from build123d import *

# Parameters (mm, degrees)
CYLINDER_R        = 3.25
CYLINDER_DEPTH    = 3.5
BOX017_W          = 43
BOX017_H          = 38
BOX017_DEPTH      = 0.5
BOX057_W          = 4
BOX057_H          = 8
BOX057_DEPTH      = 5.3
BOX001_W          = 4.5
BOX001_H          = 2.5
BOX001_DEPTH      = 5.3
BOX003_W          = 5.5
BOX003_H          = 3.5
BOX003_DEPTH      = 5.3
BOX002_W          = 53.8
BOX002_H          = 62.8
BOX002_DEPTH      = 5.3
BOX_W             = 56.3
BOX_H             = 64.25
BOX_DEPTH         = 5.3
BOX056_W          = 13.5
BOX056_H          = 1
BOX056_DEPTH      = 5
BOX041_W          = 44
BOX041_H          = 39
BOX041_DEPTH      = 0.5
BOX008_W          = 56.3
BOX008_H          = 39
BOX008_DEPTH      = 2
CHAMFER_SIZE      = 1.5
CYLINDER011_R     = 5
CYLINDER011_DEPTH = 0.5
BOX055_W          = 32
BOX055_H          = 10
BOX055_DEPTH      = 0.5
CYLINDER010_R     = 5
CYLINDER010_DEPTH = 0.5
BOX044_W          = 32
BOX044_H          = 12
BOX044_DEPTH      = 1
CYLINDER007_R     = 6
CYLINDER007_DEPTH = 1
CYLINDER006_R     = 6
CYLINDER006_DEPTH = 1
CYLINDER008_R     = 7
CYLINDER008_DEPTH = 1
BOX047_W          = 10
BOX047_H          = 1
BOX047_DEPTH      = 1
BOX049_W          = 10
BOX049_H          = 1
BOX049_DEPTH      = 1
BOX048_W          = 10
BOX048_H          = 1
BOX048_DEPTH      = 1
BOX046_W          = 10
BOX046_H          = 1
BOX046_DEPTH      = 1
BOX045_W          = 10
BOX045_H          = 1
BOX045_DEPTH      = 1
CYLINDER009_R     = 7
CYLINDER009_DEPTH = 1
BOX051_W          = 10
BOX051_H          = 1
BOX051_DEPTH      = 1
BOX054_W          = 10
BOX054_H          = 1
BOX054_DEPTH      = 1
BOX053_W          = 10
BOX053_H          = 1
BOX053_DEPTH      = 1
BOX052_W          = 10
BOX052_H          = 1
BOX052_DEPTH      = 1
BOX050_W          = 10
BOX050_H          = 1
BOX050_DEPTH      = 1
BOX010_W          = 10
BOX010_H          = 10
BOX010_DEPTH      = 10
BOX007_W          = 56.3
BOX007_H          = 25.25
BOX007_DEPTH      = 2


with BuildPart() as cylinder_magnet:
    # Cylinder → Cylinder (new body)
    with BuildSketch(Plane(origin=(52.8, 32.25, 3.7), x_dir=(0, 0, -1), z_dir=(1, 0, 0))):
        Circle(CYLINDER_R)
    extrude(amount=CYLINDER_DEPTH)


with BuildPart() as obj1:
    # Box017 → Box017 (new body)
    with BuildSketch(Plane(origin=(7.1, 8.5, 6.8), x_dir=(1, 0, 0), z_dir=(0, 0, 1))):
        with Locations((21.5, 19)):
            Rectangle(BOX017_W, BOX017_H)
    extrude(amount=BOX017_DEPTH)


with BuildPart() as cube_magnet_black:
    # Box057 → Box057 (new body)
    with BuildSketch(Plane(origin=(51.3, 28.25, 0), x_dir=(1, 0, 0), z_dir=(0, 0, 1))):
        with Locations((2, 4)):
            Rectangle(BOX057_W, BOX057_H)
    extrude(amount=BOX057_DEPTH)


with BuildPart() as cube_corner_inner:
    # Box001 → Box001 (new body)
    with BuildSketch(Plane(origin=(51.8, 61.75, 0), x_dir=(1, 0, 0), z_dir=(0, 0, 1))):
        with Locations((2.25, 1.25)):
            Rectangle(BOX001_W, BOX001_H)
    extrude(amount=BOX001_DEPTH)


with BuildPart() as cube_corner_outer:
    # Box003 → Box003 (new body)
    with BuildSketch(Plane(origin=(50.8, 60.75, 0), x_dir=(1, 0, 0), z_dir=(0, 0, 1))):
        with Locations((2.75, 1.75)):
            Rectangle(BOX003_W, BOX003_H)
    extrude(amount=BOX003_DEPTH)


with BuildPart() as cube_inner_base:
    # Box002 → Box002 (new body)
    with BuildSketch(Plane(origin=(1.25, 0, 0), x_dir=(1, 0, 0), z_dir=(0, 0, 1))):
        with Locations((26.9, 31.4)):
            Rectangle(BOX002_W, BOX002_H)
    extrude(amount=BOX002_DEPTH)


with BuildPart() as cut024:
    # Box → Box (new body)
    with BuildSketch(Plane.XY):
        with Locations((28.15, 32.125)):
            Rectangle(BOX_W, BOX_H)
    extrude(amount=BOX_DEPTH)

    # Cut: cut Cube(inner_base)
    add(cube_inner_base.part, mode=Mode.SUBTRACT)

    # Fusion: union Cube(corner_outer)
    add(cube_corner_outer.part)

    # Cut024: cut Cube(corner_inner)
    add(cube_corner_inner.part, mode=Mode.SUBTRACT)


with BuildPart() as cube_sd_card_cover:
    # Box056 → Box056 (new body)
    with BuildSketch(Plane(origin=(27.1, 63.25, -5), x_dir=(1, 0, 0), z_dir=(0, 0, 1))):
        with Locations((6.75, 0.5)):
            Rectangle(BOX056_W, BOX056_H)
    extrude(amount=BOX056_DEPTH)


with BuildPart() as obj2:
    # Box041 → Box041 (new body)
    with BuildSketch(Plane(origin=(6.6, 8, 6.8), x_dir=(1, 0, 0), z_dir=(0, 0, 1))):
        with Locations((22, 19.5)):
            Rectangle(BOX041_W, BOX041_H)
    extrude(amount=BOX041_DEPTH)


with BuildPart() as chamfer_body:
    # Box008 → Box008 (new body)
    with BuildSketch(Plane.XY.offset(5.3)):
        with Locations((28.15, 19.5)):
            Rectangle(BOX008_W, BOX008_H)
    extrude(amount=BOX008_DEPTH)

    # Chamfer
    chamfer_edges = [chamfer_body.edges().sort_by_distance(p)[0] for p in [
        (0, 19.5, 7.3),
        (56.3, 19.5, 7.3),
    ]]
    chamfer(chamfer_edges, length=CHAMFER_SIZE)


with BuildPart() as cylinder002_right_nintendo_inner:
    # Cylinder011 → Cylinder011 (new body)
    with BuildSketch(Plane(origin=(44.6, 55, 6.8), x_dir=(1, 0, 0), z_dir=(0, 0, 1))):
        Circle(CYLINDER011_R)
    extrude(amount=CYLINDER011_DEPTH)


with BuildPart() as cube_middle_nintendo_inner:
    # Box055 → Box055 (new body)
    with BuildSketch(Plane(origin=(12.6, 50, 6.8), x_dir=(1, 0, 0), z_dir=(0, 0, 1))):
        with Locations((16, 5)):
            Rectangle(BOX055_W, BOX055_H)
    extrude(amount=BOX055_DEPTH)


with BuildPart() as fusion033:
    # Cylinder010 → Cylinder010 (new body)
    with BuildSketch(Plane(origin=(12.6, 55, 6.8), x_dir=(1, 0, 0), z_dir=(0, 0, 1))):
        Circle(CYLINDER010_R)
    extrude(amount=CYLINDER010_DEPTH)

    # Fusion033: union Cylinder002(right_nintendo_inner), Cube(middle_nintendo_inner)
    add(cylinder002_right_nintendo_inner.part)
    add(cube_middle_nintendo_inner.part)


with BuildPart() as cube_middle_nintendo_outer:
    # Box044 → Box044 (new body)
    with BuildSketch(Plane(origin=(12.6, 49, 6.8), x_dir=(1, 0, 0), z_dir=(0, 0, 1))):
        with Locations((16, 6)):
            Rectangle(BOX044_W, BOX044_H)
    extrude(amount=BOX044_DEPTH)


with BuildPart() as cylinder002_right_nintendo_outer:
    # Cylinder007 → Cylinder007 (new body)
    with BuildSketch(Plane(origin=(44.6, 55, 6.8), x_dir=(1, 0, 0), z_dir=(0, 0, 1))):
        Circle(CYLINDER007_R)
    extrude(amount=CYLINDER007_DEPTH)


with BuildPart() as cylinder001_left_nintendo_outer:
    # Cylinder006 → Cylinder006 (new body)
    with BuildSketch(Plane(origin=(12.6, 55, 6.8), x_dir=(1, 0, 0), z_dir=(0, 0, 1))):
        Circle(CYLINDER006_R)
    extrude(amount=CYLINDER006_DEPTH)


with BuildPart() as cylinder001_left_nintendo_fin_cut:
    # Cylinder008 → Cylinder008 (new body)
    with BuildSketch(Plane(origin=(12.6, 55, 6.8), x_dir=(1, 0, 0), z_dir=(0, 0, 1))):
        Circle(CYLINDER008_R)
    extrude(amount=CYLINDER008_DEPTH)


with BuildPart() as box047:
    # Box047 → Box047 (new body)
    with BuildSketch(Plane(origin=(0, 54.5, 6.8), x_dir=(1, 0, 0), z_dir=(0, 0, 1))):
        with Locations((5, 0.5)):
            Rectangle(BOX047_W, BOX047_H)
    extrude(amount=BOX047_DEPTH)


with BuildPart() as box049:
    # Box049 → Box049 (new body)
    with BuildSketch(Plane(origin=(0, 58.5, 6.8), x_dir=(1, 0, 0), z_dir=(0, 0, 1))):
        with Locations((5, 0.5)):
            Rectangle(BOX049_W, BOX049_H)
    extrude(amount=BOX049_DEPTH)


with BuildPart() as box048:
    # Box048 → Box048 (new body)
    with BuildSketch(Plane(origin=(0, 56.5, 6.8), x_dir=(1, 0, 0), z_dir=(0, 0, 1))):
        with Locations((5, 0.5)):
            Rectangle(BOX048_W, BOX048_H)
    extrude(amount=BOX048_DEPTH)


with BuildPart() as box046:
    # Box046 → Box046 (new body)
    with BuildSketch(Plane(origin=(0, 52.5, 6.8), x_dir=(1, 0, 0), z_dir=(0, 0, 1))):
        with Locations((5, 0.5)):
            Rectangle(BOX046_W, BOX046_H)
    extrude(amount=BOX046_DEPTH)


with BuildPart() as cut009:
    # Box045 → Box045 (new body)
    with BuildSketch(Plane(origin=(0, 50.5, 6.8), x_dir=(1, 0, 0), z_dir=(0, 0, 1))):
        with Locations((5, 0.5)):
            Rectangle(BOX045_W, BOX045_H)
    extrude(amount=BOX045_DEPTH)

    # Fusion004: union Box047, Box049, Box048, Box046
    add(box047.part)
    add(box049.part)
    add(box048.part)
    add(box046.part)

    # Cut009: cut Cylinder001(left_nintendo_fin_cut)
    add(cylinder001_left_nintendo_fin_cut.part, mode=Mode.SUBTRACT)


with BuildPart() as cylinder002_right_nintendo_fin_cut:
    # Cylinder009 → Cylinder009 (new body)
    with BuildSketch(Plane(origin=(44.6, 55, 6.8), x_dir=(1, 0, 0), z_dir=(0, 0, 1))):
        Circle(CYLINDER009_R)
    extrude(amount=CYLINDER009_DEPTH)


with BuildPart() as box051:
    # Box051 → Box051 (new body)
    with BuildSketch(Plane(origin=(46.3, 54.5, 6.8), x_dir=(1, 0, 0), z_dir=(0, 0, 1))):
        with Locations((5, 0.5)):
            Rectangle(BOX051_W, BOX051_H)
    extrude(amount=BOX051_DEPTH)


with BuildPart() as box054:
    # Box054 → Box054 (new body)
    with BuildSketch(Plane(origin=(46.3, 52.5, 6.8), x_dir=(1, 0, 0), z_dir=(0, 0, 1))):
        with Locations((5, 0.5)):
            Rectangle(BOX054_W, BOX054_H)
    extrude(amount=BOX054_DEPTH)


with BuildPart() as box053:
    # Box053 → Box053 (new body)
    with BuildSketch(Plane(origin=(46.3, 56.5, 6.8), x_dir=(1, 0, 0), z_dir=(0, 0, 1))):
        with Locations((5, 0.5)):
            Rectangle(BOX053_W, BOX053_H)
    extrude(amount=BOX053_DEPTH)


with BuildPart() as box052:
    # Box052 → Box052 (new body)
    with BuildSketch(Plane(origin=(46.3, 58.5, 6.8), x_dir=(1, 0, 0), z_dir=(0, 0, 1))):
        with Locations((5, 0.5)):
            Rectangle(BOX052_W, BOX052_H)
    extrude(amount=BOX052_DEPTH)


with BuildPart() as cut008:
    # Box050 → Box050 (new body)
    with BuildSketch(Plane(origin=(46.3, 50.5, 6.8), x_dir=(1, 0, 0), z_dir=(0, 0, 1))):
        with Locations((5, 0.5)):
            Rectangle(BOX050_W, BOX050_H)
    extrude(amount=BOX050_DEPTH)

    # Fusion003: union Box051, Box054, Box053, Box052
    add(box051.part)
    add(box054.part)
    add(box053.part)
    add(box052.part)

    # Cut008: cut Cylinder002(right_nintendo_fin_cut)
    add(cylinder002_right_nintendo_fin_cut.part, mode=Mode.SUBTRACT)


with BuildPart() as cube_top_corner_cut:
    # Box010 → Box010 (new body)
    with BuildSketch(Plane(origin=(51.8, 61.75, 0), x_dir=(1, 0, 0), z_dir=(0, 0, 1))):
        with Locations((5, 5)):
            Rectangle(BOX010_W, BOX010_H)
    extrude(amount=BOX010_DEPTH)


with BuildPart() as cut026:
    # Box007 → Box007 (new body)
    with BuildSketch(Plane(origin=(0, 39, 5.3), x_dir=(1, 0, 0), z_dir=(0, 0, 1))):
        with Locations((28.15, 12.625)):
            Rectangle(BOX007_W, BOX007_H)
    extrude(amount=BOX007_DEPTH)

    # Cut006: cut Cube(top_corner_cut)
    add(cube_top_corner_cut.part, mode=Mode.SUBTRACT)

    # Cut010: cut Cut008
    add(cut008.part, mode=Mode.SUBTRACT)

    # Cut011: cut Cut009
    add(cut009.part, mode=Mode.SUBTRACT)

    # Cut012: cut Cylinder001(left_nintendo_outer)
    add(cylinder001_left_nintendo_outer.part, mode=Mode.SUBTRACT)

    # Cut013: cut Cylinder002(right_nintendo_outer)
    add(cylinder002_right_nintendo_outer.part, mode=Mode.SUBTRACT)

    # Cut014: cut Cube(middle_nintendo_outer)
    add(cube_middle_nintendo_outer.part, mode=Mode.SUBTRACT)

    # Fusion034: union Chamfer body, Fusion033
    add(chamfer_body.part)
    add(fusion033.part)

    # Cut025: cut obj2)
    add(obj2.part, mode=Mode.SUBTRACT)

    # Fusion035: union obj1), Cube(magnet_black), Cut024, Cube(sd_card_cover)
    add(obj1.part)
    add(cube_magnet_black.part)
    add(cut024.part)
    add(cube_sd_card_cover.part)

    # Cut026: cut Cylinder(magnet)
    add(cylinder_magnet.part, mode=Mode.SUBTRACT)


solid = cut026.part
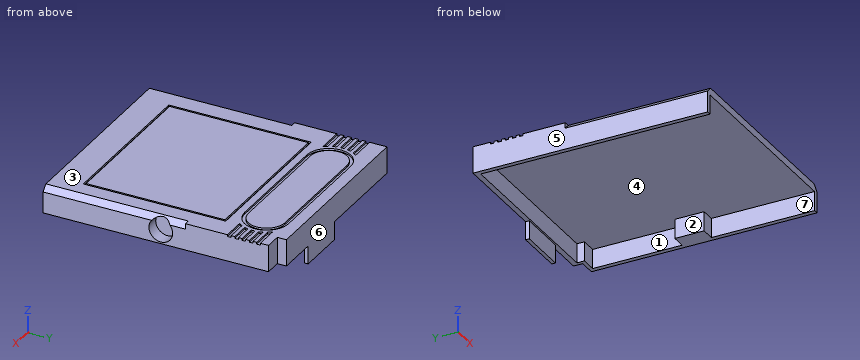
Check sheet for the modelled part. Datum: model origin and axes. Units: mm. Face numbers are marked on the shaded views. A direction names the side the tool comes from. Round coordinates to 2 decimals unless told otherwise and drop trailing zeros. Order: outer loops, then holes, each group sorted by start corner. A loop starts at its lowest first (then second) coordinate and runs counter-clockwise, first axis right, second up.
(1) Cross-section at B-B, the plane x = 32. Enter the section's corners in (y, z), and give its area (3 significant figures).
(2) Cross-section at D-D, the plane y = 26. Enter the section's corners in (x, z), and give its area (3 significant figures).
(3) Cross-section at A-A, the plane z = 4.5. Enter the section's corners in (x, y).
(4) Cross-section at C-C, the plane y = 6. Enter the section's corners in (x, z).
(5) Scan lines: probe 1 along Z at (x, y) = (53.9, 32.25); probe 2 along Y at (x, z) = (54.25, 3.7); probe 3 along X at (y, z) = (17.5, 2). Record each from-to range of solid material in increasing order.
(6) Access from +Z, -Z, +X, -X, +Y, -Y to the whole of each face (thin tool, end or side, straight path). Record for the marked faces 1, 2 and 3.
(7) Draft check along X on the marked faces 4, 5, 6 and 7. Enter one of: pulls with the +X half, pulls with the -X half, needs draft (parallel to the pull), parting line crosses it, or undercut.
(8) Go/stop test with flat-tipped pins: P1, Ø2, axis at x = 16, y = 33, coming from the -Z side; P2, Ø0.6, axis at x = 55, z = 7, coming from the -Y side; P3, Ø4, axis at x = 50.5, z = 1.5, coming from the -Y side; P4, Ø1.6, axis at x = 28, z = 3, coming from the -Y side. Record where each tip stops, or that it passes through.
Check sheet entries:
1. outline: (0, 5.3) - (62.8, 5.3) - (62.8, 0) - (63.25, 0) - (63.25, -5) - (64.25, -5) - (64.25, 7.3) - (61, 7.3) - (61, 6.8) - (60, 6.8) - (60, 7.3) - (50, 7.3) - (50, 6.8) - (49, 6.8) - (49, 7.3) - (47, 7.3) - (47, 6.8) - (46.5, 6.8) - (46.5, 7.3) - (8.5, 7.3) - (8.5, 6.8) - (8, 6.8) - (8, 7.3) - (0, 7.3) - close
1. area: 140 mm2
2. outline: (0, 0) - (1.25, 0) - (1.25, 5.3) - (55.05, 5.3) - (55.05, 0) - (56.3, 0) - (56.3, 5.8) - (54.8, 7.3) - (50.6, 7.3) - (50.6, 6.8) - (50.1, 6.8) - (50.1, 7.3) - (7.1, 7.3) - (7.1, 6.8) - (6.6, 6.8) - (6.6, 7.3) - (1.5, 7.3) - (0, 5.8) - close
2. area: 123 mm2
3. outline: (0, 0) - (1.25, 0) - (1.25, 62.8) - (50.8, 62.8) - (50.8, 60.75) - (55.05, 60.75) - (55.05, 36.25) - (51.3, 36.25) - (51.3, 28.25) - (55.05, 28.25) - (55.05, 0) - (56.3, 0) - (56.3, 29.1) - (52.8, 29.1) - (52.8, 35.4) - (56.3, 35.4) - (56.3, 61.75) - (51.8, 61.75) - (51.8, 64.25) - (0, 64.25) - close
4. outline: (0, 0) - (1.25, 0) - (1.25, 5.3) - (55.05, 5.3) - (55.05, 0) - (56.3, 0) - (56.3, 5.8) - (54.8, 7.3) - (1.5, 7.3) - (0, 5.8) - close
5. probe 1: z = 0 to 0.45, 6.95 to 7.3
5. probe 2: y = 28.25 to 29, 35.5 to 36.25, 60.75 to 61.75
5. probe 3: x = 0 to 1.25, 55.05 to 56.3
6. face 1: -Z
6. face 2: -Z, -Y
6. face 3: +Z, +X, -X, +Y, -Y
7. face 4: undercut
7. face 5: pulls with the -X half
7. face 6: needs draft
7. face 7: undercut
8. P1: stops at z = 5.3
8. P2: stops at y = 0
8. P3: stops at y = 28.25
8. P4: stops at y = 62.8
